For this review, use the dimensioned drawing (mm, ordinates from the lowest corner) and the shaded views. Give positions to 0.01 mm unless a question says otherwise; leave off trailing zeros. Write each loop counter-clockwise with the first axis right and the second up, starting at its lowest first coordinate (ties: lowest second). Pieces come first, ordered by that corner, then holes. Notation, with made-up numbers: (-22.75, 15.25) -> (3.25, 15.25) arc R28 ccw to (3.25, 42.25) -> close; hole circle Ø2 at (30, 67.25). An arc over 180 degrees is marked (long way). Answer as CSV lines item,"result".
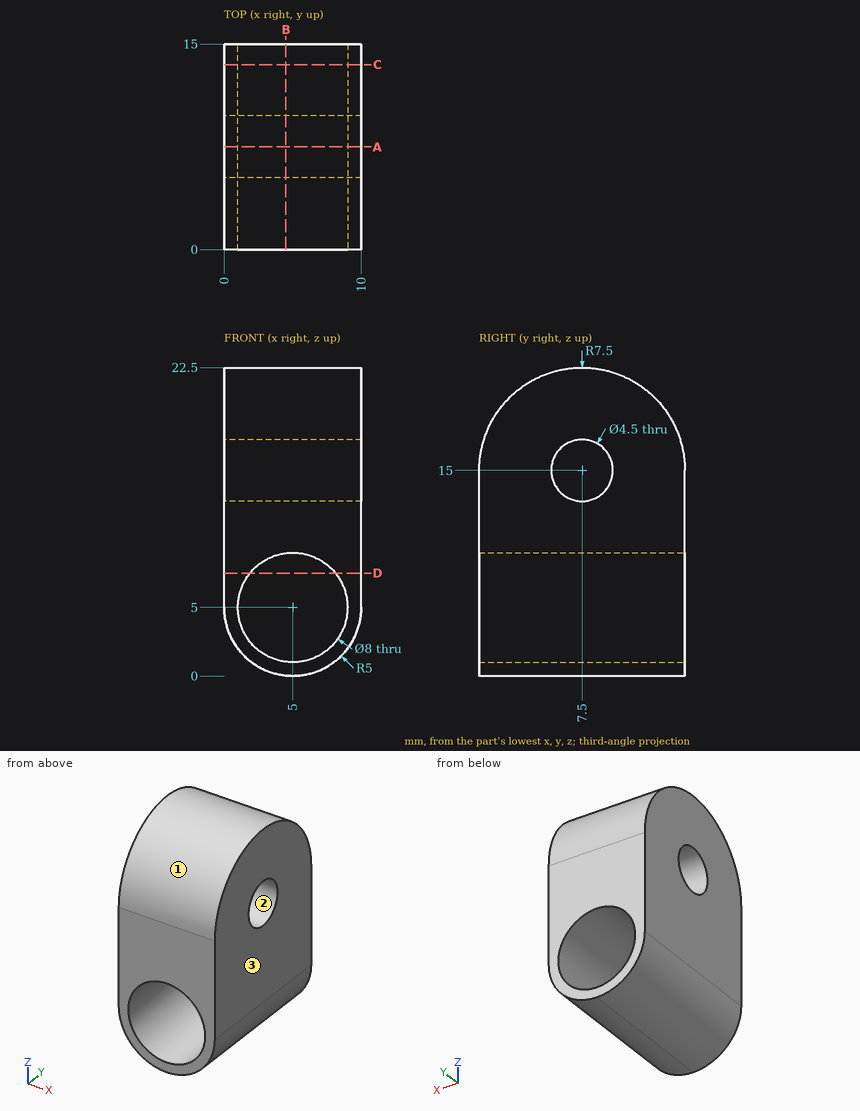
Q1. Clearance check with flat-ended pins moving along their axes: pin 1 (6 mm diameter, centred on x = 2.5, y = 8, fed in from -Z); pin 2 (1 mm diameter, centred on x = 1.5, z = 19, fed in from +Y). State where each tip first meets the part, or that it passes through.
Answer block:
pin 1,"stops at z = 0"
pin 2,"stops at y = 14.13"
Q2. Add section C-C (y = 13.5). Write out the cut boundary in (x, z).
Answer block:
outline,"(0, 5) arc R5 ccw to (10, 5) -> (10, 19.5) -> (0, 19.5) -> close; hole circle Ø8 at (5, 5)"
Q3. Add section B-B (x = 4.5). Write out the cut boundary in (y, z).
Answer block:
outline,"(0, 0.03) -> (15, 0.03) -> (15, 1.03) -> (0, 1.03) -> close; (0, 8.97) -> (15, 8.97) -> (15, 15) arc R7.5 ccw to (0, 15) -> close; hole circle Ø4.5 at (7.5, 15)"
Q4. To check wall thickness, follow probe 1 along Z at (x, y) = (8.5, 7.25); probe 2 along Y at (x, z) = (6, 15); probe 3 along Z at (x, y) = (5, 9.5). State the ranges of each line that lie inside material, in increasing order. Write a range as [from, to].
Answer block:
probe 1,"z = [1.43, 3.06], [6.94, 12.76], [17.24, 22.5]"
probe 2,"y = [0, 5.25], [9.75, 15]"
probe 3,"z = [0, 1], [9, 13.97], [16.03, 22.23]"
Q5. Add section A-A (y = 7.5). Write out the cut boundary in (x, z).
Answer block:
outline,"(0, 5) arc R5 ccw to (10, 5) -> (10, 12.75) -> (0, 12.75) -> close; (0, 17.25) -> (10, 17.25) -> (10, 22.5) -> (0, 22.5) -> close; hole circle Ø8 at (5, 5)"
Q6. Add section D-D (z = 7.5). Write out the cut boundary in (x, y).
Answer block:
outline,"(0, 0) -> (1.88, 0) -> (1.88, 15) -> (0, 15) -> close; (8.12, 0) -> (10, 0) -> (10, 15) -> (8.12, 15) -> close"
Q7. Draft analysis for pull direction Z (two halves, no side actions). For the marked faces 1, 2 and 3, state which applies: released by +Z, released by -Z, zero draft, split by the parting line, or undercut.
Answer block:
face 1,"released by +Z"
face 2,"undercut"
face 3,"zero draft"
